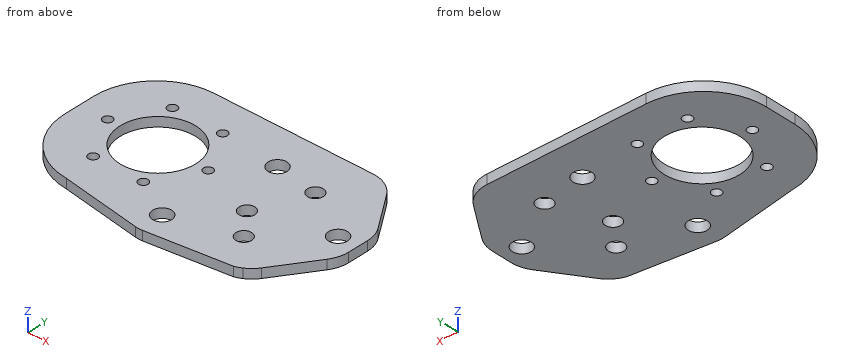
```python
from build123d import *

# Parameters (mm, degrees)
ESBO_O1_W                = 76
ESBO_O1_H                = 50
ESBO_O1_R                = 2.5
ESBO_O1_R_2              = 12
ESBO_O1_R_3              = 1.5
RESSALTO_EXTRUS_O1_DEPTH = 3
ESBO_O2_R                = 2.5
CORTE_EXTRUS_O1_DEPTH    = 3
FILETE1_R                = 20
ESBO_O3_R                = 2.5
RESSALTO_EXTRUS_O2_DEPTH = 3
ESBO_O5_R                = 3
CORTE_EXTRUS_O2_DEPTH    = 92.021975369
RESSALTO_EXTRUS_O3_DEPTH = 3
RESSALTO_EXTRUS_O4_DEPTH = 3
FILETE2_R                = 10
ESBO_O7_R                = 2.5
CORTE_EXTRUS_O3_DEPTH    = 10


with BuildPart() as part:
    # Esboço1 → Ressalto-extrusão1 (new body)
    with BuildSketch(Plane.XY):
        with Locations((38, 25)):
            Rectangle(ESBO_O1_W, ESBO_O1_H)
        with Locations((59.25, 18.5)):
            Circle(ESBO_O1_R, mode=Mode.SUBTRACT)
        with Locations((25, 25)):
            Circle(ESBO_O1_R_2, mode=Mode.SUBTRACT)
        with Locations((17, 38.856406461)):
            Circle(ESBO_O1_R_3, mode=Mode.SUBTRACT)
        with Locations((33, 38.856406461)):
            Circle(ESBO_O1_R_3, mode=Mode.SUBTRACT)
        with Locations((41, 25)):
            Circle(ESBO_O1_R_3, mode=Mode.SUBTRACT)
        with Locations((33, 11.143593539)):
            Circle(ESBO_O1_R_3, mode=Mode.SUBTRACT)
        with Locations((17, 11.143593539)):
            Circle(ESBO_O1_R_3, mode=Mode.SUBTRACT)
        with Locations((9, 25)):
            Circle(ESBO_O1_R_3, mode=Mode.SUBTRACT)
    extrude(amount=RESSALTO_EXTRUS_O1_DEPTH)

    # Esboço2 → Corte-extrusão1 (cut)
    with BuildSketch(Plane.XY.offset(3)):
        with Locations((66, 35)):
            Circle(ESBO_O2_R)
        with Locations((66, 15)):
            Circle(ESBO_O2_R)
    extrude(amount=-CORTE_EXTRUS_O1_DEPTH, mode=Mode.SUBTRACT)

    # Filete1
    filete1_edges = [part.edges().sort_by_distance(p)[0] for p in [
        (0, 50, 1.5),
        (0, 0, 1.5),
    ]]
    fillet(filete1_edges, radius=FILETE1_R)

    # Esboço3 → Ressalto-extrusão2 (add, through all)
    with BuildSketch(Plane.XY.offset(3)):
        with Locations((66, 15)):
            Circle(ESBO_O3_R)
        with Locations((66, 35)):
            Circle(ESBO_O3_R)
    extrude(amount=-RESSALTO_EXTRUS_O2_DEPTH)

    # Esboço5 → Corte-extrusão2 (cut, through all)
    with BuildSketch(Plane(origin=(0, 0, 0), x_dir=(-1, 0, 0), z_dir=(0, 0, -1))):
        with Locations((-45.680731562, 3.807316308)):
            Circle(ESBO_O5_R)
        with Locations((-52.0071049, 37.142437356)):
            Circle(ESBO_O5_R)
    extrude(amount=-CORTE_EXTRUS_O2_DEPTH, mode=Mode.SUBTRACT)

    # Esboço4 → Ressalto-extrusão3 (add, through all)
    with BuildSketch(Plane(origin=(0, 0, 0), x_dir=(-1, 0, 0), z_dir=(0, 0, -1))):
        with BuildLine():
            ThreePointArc((-18.605557994, 0.048670934), (-19.30235443, 0.012171437), (-20, 0))
            Line((-20, 0), (-74.805369877, 0))
            ThreePointArc((-74.805369877, 0), (-73.762195737, -0.525177263), (-72.66490464, -0.925146879))
            Line((-72.66490464, -0.925146879), (-46.660572258, -4.133783454))
            ThreePointArc((-46.660572258, -4.133783454), (-45.535290053, -4.192683692), (-44.412892385, -4.09292021))
            Line((-44.412892385, -4.09292021), (-18.605557994, 0.048670934))
        make_face()
    extrude(amount=-RESSALTO_EXTRUS_O3_DEPTH)

    # Esboço6 → Ressalto-extrusão4 (add, through all)
    with BuildSketch(Plane.XY.offset(3)):
        with BuildLine():
            Line((88.7, 31.35), (76, 50))
            Line((76, 50), (76, 25))
            Line((76, 25), (79.35, 25))
            ThreePointArc((79.35, 25), (82.35, 28), (85.35, 25))
            Line((85.35, 25), (88.7, 25))
            Line((88.7, 25), (88.7, 31.35))
        make_face()
        with BuildLine():
            Line((79.35, 25), (76, 25))
            Line((76, 25), (76, 0))
            Line((76, 0), (88.7, 18.65))
            Line((88.7, 18.65), (88.7, 25))
            Line((88.7, 25), (85.35, 25))
            ThreePointArc((85.35, 25), (82.35, 22), (79.35, 25))
        make_face()
    extrude(amount=-RESSALTO_EXTRUS_O4_DEPTH)

    # Filete2
    # the kernel refuses this fillet: 10 mm, written as the material it takes off along each edge
    with BuildSketch(Plane(origin=(88.7, 18.65, 10.703782372), x_dir=(-0.5628554049483921, -0.8265553781328759, 0), z_dir=(0, 0, -1)), Plane(origin=(88.7, 31.35, 10.703782372), x_dir=(0, -1, 0), z_dir=(0, 0, -1))) as filete2_piece_1:
        with BuildLine():
            CenterArc((FILETE2_R * 0.308151294884, FILETE2_R), FILETE2_R, 235.746501053, 34.253498947)
            Line((-FILETE2_R * 0.254704110065, FILETE2_R * 0.173444621867), (-FILETE2_R * 0.265961218164, FILETE2_R * 0.156913514304))
            Line((-FILETE2_R * 0.265961218164, FILETE2_R * 0.156913514304), (-FILETE2_R * 0.00616302589767, -FILETE2_R * 0.02))
            Line((-FILETE2_R * 0.00616302589767, -FILETE2_R * 0.02), (FILETE2_R * 0.308151294884, -FILETE2_R * 0.02))
            Line((FILETE2_R * 0.308151294884, -FILETE2_R * 0.02), (FILETE2_R * 0.308151294884, 0))
        make_face()
    extrude(amount=18.407564744, mode=Mode.SUBTRACT)
    with BuildSketch(Plane(origin=(76, 50, -13.221878613), x_dir=(-1, 0, 0), z_dir=(0, 0, 1))) as filete2_piece_2:
        with BuildLine():
            CenterArc((FILETE2_R * 0.528875144505, FILETE2_R), FILETE2_R, 214.253498947, 55.746501053)
            Line((-FILETE2_R * 0.297680233628, FILETE2_R * 0.437144595052), (-FILETE2_R * 0.31421134119, FILETE2_R * 0.425887486953))
            Line((-FILETE2_R * 0.31421134119, FILETE2_R * 0.425887486953), (-FILETE2_R * 0.0105775028901, -FILETE2_R * 0.02))
            Line((-FILETE2_R * 0.0105775028901, -FILETE2_R * 0.02), (FILETE2_R * 0.528875144505, -FILETE2_R * 0.02))
            Line((FILETE2_R * 0.528875144505, -FILETE2_R * 0.02), (FILETE2_R * 0.528875144505, 0))
        make_face()
    extrude(amount=29.443757225, mode=Mode.SUBTRACT)
    with BuildSketch(Plane(origin=(76, 0, -9.151102244), x_dir=(-1, 0, 0), z_dir=(0, 0, 1))) as filete2_piece_3:
        with BuildLine():
            CenterArc((6.205254838, -8.65411116), FILETE2_R, 120.070317479, 25.676183574)
            Line((-2.060298944, -3.02555711), (-2.225610019, -2.912986029))
            Line((-2.225610019, -2.912986029), (-0.165311076, 0.112571081))
            Line((-0.165311076, 0.112571081), (0, 0.2))
            ThreePointArc((0, 0.2), (0.597315061, 0.2), (1.094417628, 0.173082223))
            Line((1.094417628, 0.173082223), (1.194630123, 0))
        make_face()
    extrude(amount=21.302204488, mode=Mode.SUBTRACT)

    # Esboço7 → Corte-extrusão3 (cut)
    with BuildSketch(Plane.XY.offset(3)):
        with Locations((66, 35)):
            Circle(ESBO_O7_R)
        with Locations((66, 10)):
            Circle(ESBO_O7_R)
    extrude(amount=-CORTE_EXTRUS_O3_DEPTH, mode=Mode.SUBTRACT)


solid = part.part
```
The listing builds one solid part. Answer for the finished solid, in the listing's coordinates (mm). Coordinates: 2 decimals unless noted, no trailing zeros. Write each loop counter-clockwise with the first axis right and the second up, starting at its lowest first coordinate (ties: lowest second). Pieces come first, ordered by that corner, then holes. Notation, with made-up numbers: (57, 52) - (74, 52) arc R33 cw to (74, 91) - close; hole circle Ø3 at (9, -1). An arc over 180 degrees is marked (long way). Return JSON: item names as keys, results as strings. Group by question number.
1. A cutting plane is placed at A-A, the plane x = 26.5. Determine the outline of the cut face in (y, z), plus the area to 3 significant figures.
2. A cutting plane is placed at B-B, the plane y = 18.5. Determine the outline of the cut face in (x, z), plus the area to 3 significant figures.
3. Given pin 1 (1.5 mm diameter, centred on y = 1.5, z = 2.5, fed in from -X), flat-ended and moving along its own axis, determine where the tip first touches the part or whether it passes through.
4. A cutting plane is placed at D-D, the plane x = 66. Determine the outline of the cut face in (y, z).
5. Straight lines are drawn through the part: L1, parallel to Y at x = 33, z = 2.35; L2, parallel to Y at x = 80.5, z = 2.85; L3, parallel to X at y = 27.5, z = 2.65. For each, find the intervals that lie inside material, in ascending order.
6. A cutting plane is placed at C-C, the plane z = 0.85. Give the number of separate pieces and of enclosed holes in the cut face, plus the area to 3 significant figures.
Ans:
{
 "1": {"outline": "(-1.22, 0) - (13.09, 0) - (13.09, 3) - (-1.22, 3) - close; (36.91, 0) - (50, 0) - (50, 3) - (36.91, 3) - close", "area": "82.2 mm²"},
 "2": {"outline": "(0.06, 0) - (14.91, 0) - (14.91, 3) - (0.06, 3) - close; (35.09, 0) - (56.75, 0) - (56.75, 3) - (35.09, 3) - close; (61.75, 0) - (88.16, 0) - (88.16, 3) - (61.75, 3) - close", "area": "189 mm²"},
 "3": {"pin 1": "x = 10.78"},
 "4": {"outline": "(-1.75, 0) - (7.5, 0) - (7.5, 3) - (-1.75, 3) - close; (12.5, 0) - (32.5, 0) - (32.5, 3) - (12.5, 3) - close; (37.5, 0) - (50, 0) - (50, 3) - (37.5, 3) - close"},
 "5": {"L1": "-2.26 to 9.64, 12.64 to 16.06, 33.94 to 37.36, 40.36 to 50", "L2": "6.61 to 22.64, 27.36 to 43.39", "L3": "0 to 13.26, 36.74 to 80.69, 84.01 to 88.7"},
 "6": {"separate pieces": "1", "enclosed holes": "13", "area": "3,510 mm²"}
}
